```python
from build123d import *

# Parameters (mm, degrees)
F0_W     = 95.948249
F0_H     = 89.254186
F0_R     = 22.222856
F1_DEPTH = 25.4
F0_R_2   = 16.979285
F2_DEPTH = 38.1
F4_DEPTH = 558.8
F5_R     = 10.492491
F5_R_2   = 10.165453
F6_DEPTH = 48.931418


with BuildPart() as f1:
    # F0 (on Front) → F1 (new body, symmetric)
    with BuildSketch(Plane.XZ):
        with Locations((-0.956293, 0.956297)):
            Rectangle(F0_W, F0_H)
        Circle(F0_R, mode=Mode.SUBTRACT)
    extrude(amount=F1_DEPTH, both=True)

    # F0 (on Front) → F2 (join, symmetric)
    with BuildSketch(Plane.XZ):
        Circle(F0_R)
        Circle(F0_R_2, mode=Mode.SUBTRACT)
    extrude(amount=F2_DEPTH, both=True)

    # F3 (on Top) → F4 (cut, symmetric)
    with BuildSketch(Plane.XY):
        Polygon((0, 50.046094), (0, -54.508805), (60.724724, -51.321156), (64.549901, 41.439444), align=None)
    extrude(amount=F4_DEPTH, both=True, mode=Mode.SUBTRACT)

    # F5 (on Right) → F6 (cut, through all)
    with BuildSketch(Plane.YZ):
        with Locations((0, -30.9202)):
            Circle(F5_R)
        with Locations((0, 32.45692)):
            Circle(F5_R_2)
    extrude(amount=-F6_DEPTH, mode=Mode.SUBTRACT)


solid = f1.part
```
Could you check a few things on this model? Use its own coordinates, in mm. A direction names the side the tool comes from. Round coordinates to 2 decimals unless told otherwise and drop trailing zeros. Loops run counter-clockwise (first coordinate to the right, second up) from the corner with the lowest first, then second, coordinate; pieces in that order, holes last. Notation, with made-up numbers: (-6.5, 71.5) - (-0.5, 71.5) arc R15 ccw to (-0.5, 99.5) - close; hole circle Ø8 at (77, 79.5). An arc over 180 degrees is marked (long way). Answer in a Markdown table with one row per item. Add a question column.
(1) If we mould it in two halves opening along Z, with no side actions, what happens to faces 3 (the face through (-24.123, -2.275, -41.163)), 4 (the face through (-30, -25.4, 2)), 5 (the face through (-22.217, -31.839, 0.489)), 6 (the face through (-16.975, 0.533, 0.373))? For each: pulls with the +Z half, pulls with the -Z half, needs draft (parallel to the pull), parting line crosses it, or undercut.
(2) If we section it at C-C (z = 0): Please give me the cut outline in (x, y), plus the area to 3 significant figures.
(3) I need wall thicknesses on line 1 along Z through (x, y) = (-24.5, 0); line 2 along Z through (x, y) = (-12, 0); line 3 along Z through (x, y) = (-3, -1). Which ranges of each line are inside material? Lowest first, please.
(4) If we section it at B-B (x = -13): Please give me the cut outline in (y, z).
(5) For faces 1 (the face through (-25, 0, 45.583)), 2 (the face through (-22.217, 31.661, 0.489)), which set-ups out of +Z, -Z, +X, -X, +Y, -Y let a thin tool reach every point of the face, with its end or its side?
(6) If we section it at A-A (y = 0): Please give me the cut outline in (x, z).
(7) If we section it at D-D (y = 17): Please give me the cut outline in (x, z), plus the area to 3 significant figures.
(8) I'm going to push flat-ended pins straight in: pin 1 (24.5 mm diameter, centred on x = -36, z = -14, fed in from +Y); pin 2 (6 mm diameter, centred on x = -14, z = 24, fed in from -Y); pin 3 (16.5 mm diameter, centred on y = 0, z = 32.46, fed in from +X). Where does each tip first touch, or does it pass through?
Model answer:
| question | item | result |
|---|---|---|
| 1 | face 3 | undercut |
| 1 | face 4 | needs draft |
| 1 | face 5 | parting line crosses it |
| 1 | face 6 | undercut |
| 2 | outline | (-48.93, -25.4) - (-22.22, -25.4) - (-22.22, -38.1) - (-16.98, -38.1) - (-16.98, 38.1) - (-22.22, 38.1) - (-22.22, 25.4) - (-48.93, 25.4) - close |
| 2 | area | 1,760 mm² |
| 3 | line 1 | z = -43.67 to -41.41, -20.43 to 22.29, 42.62 to 45.58 |
| 3 | line 2 | z = -43.67 to -41.41, -20.43 to -12.01, 12.01 to 22.29, 42.62 to 45.58 |
| 3 | line 3 | z = -43.67 to -41.36, -20.48 to -16.71, 16.71 to 22.34, 42.57 to 45.58 |
| 4 | outline | (-38.1, -18.02) - (-25.4, -18.02) - (-25.4, -43.67) - (25.4, -43.67) - (25.4, -18.02) - (38.1, -18.02) - (38.1, -10.92) - (-38.1, -10.92) - close; (-38.1, 10.92) - (38.1, 10.92) - (38.1, 18.02) - (25.4, 18.02) - (25.4, 45.58) - (-25.4, 45.58) - (-25.4, 18.02) - (-38.1, 18.02) - close; hole circle Ø20.98 at (0, -30.92); hole circle Ø20.33 at (0, 32.46) |
| 5 | face 1 | +Z, +X, -X, +Y, -Y |
| 5 | face 2 | -X, +Y |
| 6 | outline | (-48.93, -43.67) - (0, -43.67) - (0, -41.41) - (-48.93, -41.41) - close; (-48.93, -20.43) - (0, -20.43) - (0, -16.98) arc R16.98 cw to (0, 16.98) - (0, 22.29) - (-48.93, 22.29) - close; (-48.93, 42.62) - (0, 42.62) - (0, 45.58) - (-48.93, 45.58) - close |
| 7 | outline | (-48.93, -43.67) - (0, -43.67) - (0, -16.98) arc R16.98 cw to (0, 16.98) - (0, 45.58) - (-48.93, 45.58) - close |
| 7 | area | 3,910 mm² |
| 8 | pin 1 | stops at y = 25.4 |
| 8 | pin 2 | stops at y = -25.4 |
| 8 | pin 3 | passes through |
